Here's how the part is built. I have some questions about the finished solid (model axes, mm). Face numbers are marked on the shaded views. Coordinates: 2 decimals unless noted, no trailing zeros. Write each loop counter-clockwise with the first axis right and the second up, starting at its lowest first coordinate (ties: lowest second). Pieces come first, ordered by that corner, then holes.
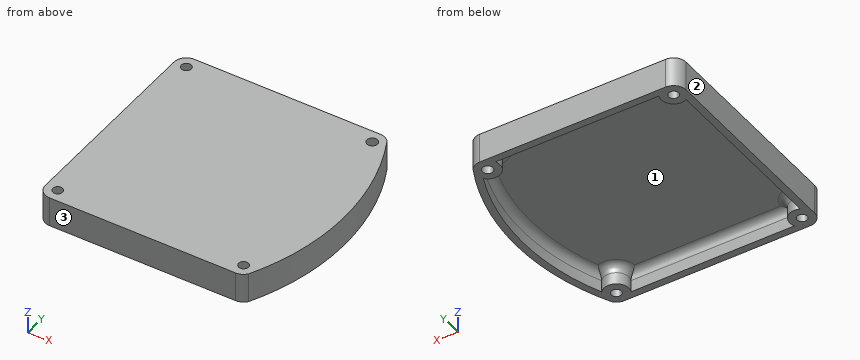
Autodesk Inventor part; units mm, degrees
ref_plane "YZ Plane" through (0, 0, 0) normal (1, 0, 0) x (0, 1, 0)
ref_plane "XZ Plane" through (0, 0, 0) normal (0, 1, 0) x (-1, 0, 0)
ref_plane "XY Plane" through (0, 0, 0) normal (0, 0, 1) x (1, 0, 0)
sketch "Sketch1" plane through (0, 0, 0) normal (0, 0, 1) x (1, 0, 0)
  line L0 (-44.1613, -40) -> (-44.1613, 40)
  arc A0 (-39.1613, 45) -> (-44.1613, 40) centre (-39.1613, 40) ccw
  line L1 (-39.1613, 45) -> (35.8387, 45)
  arc A1 (39.8387, 43) -> (35.8387, 45) centre (35.8387, 40) ccw
  arc A2 (39.8387, -43) -> (39.8387, 43) centre (-44.1612, 0) ccw
  arc A3 (35.8387, -45) -> (39.8387, -43) centre (35.8387, -39.9999) ccw
  line L2 (35.8387, -45) -> (-39.1613, -45)
  arc A4 (-44.1613, -40) -> (-39.1613, -45) centre (-39.1613, -40) ccw
  circle A5 centre (-39.1613, -40) radius 2
  circle A6 centre (-39.1613, 40) radius 2
  circle A7 centre (35.8387, 40) radius 2.15
  circle A8 centre (35.8387, -40) radius 2
  arc A9 (37.5587, 41.29) -> (35.8387, 42.15) centre (35.8387, 40) ccw
  line L3 (35.8387, 42.15) -> (-39.1613, 42.15)
  arc A10 (-39.1613, 42.15) -> (-41.3113, 40) centre (-39.1613, 40) ccw
  line L4 (-41.3113, 40) -> (-41.3113, -40)
  arc A11 (-41.3113, -40) -> (-39.1613, -42.15) centre (-39.1613, -40) ccw
  line L5 (-39.1613, -42.15) -> (35.8387, -42.15)
  arc A12 (35.8387, -42.15) -> (37.5587, -41.29) centre (35.8387, -39.9999) ccw
  arc A13 (37.3698, -41.7362) -> (37.3698, 41.7362) centre (-44.1612, 0) ccw
  circle A14 centre (-39.1613, 40) radius 5
  circle A15 centre (35.8387, 40) radius 5
  circle A16 centre (35.8387, -40) radius 5
  circle A17 centre (-39.1613, -40) radius 5
  point P0 (0, 0)
  point P1 (39.8387, -43)
  point P2 (31.3246, 42.15)
  point P3 (39.7021, 36.826)
  point P4 (39.7021, -36.826)
  point P5 (31.3246, -42.15)
  point P6 (-34.6471, -42.15)
  point P7 (-41.3113, -35.4859)
  point P8 (-41.3113, 35.4859)
  point P9 (-34.6471, 42.15)
extrude "Extrusion1" add sketch "Sketch1" along normal blind 8 contours A17 L4 A11 L5 A4 | L0 A14 L4 A17 | A0 A14 L3 A10 L4 | A17 L5 A16 L2 | A17 L5 A11 L4 | L1 A15 L3 A14 | L4 A10 L3 A14 | A16 A2 A3 | A1 A2 A15 A13 A7 L3 | L3 A7 A13 A15 | A16 A13 A15 A2
sketch "Sketch2" plane through (0, 0, 8) normal (0, 0, 1) x (1, 0, 0)
  arc A0 (-39.1613, 45) -> (-44.1613, 40) centre (-39.1613, 40) ccw
  line L0 (-44.1613, 40) -> (-44.1613, -40)
  arc A1 (-44.1613, -40) -> (-39.1613, -45) centre (-39.1613, -40) ccw
  line L1 (-39.1613, -45) -> (35.8387, -45)
  arc A2 (35.8387, -45) -> (39.8387, -43) centre (35.8387, -39.9999) ccw
  arc A3 (39.8387, -43) -> (39.8387, 43) centre (-44.1612, 0) ccw
  arc A4 (39.8387, 43) -> (35.8387, 45) centre (35.8387, 40) ccw
  line L2 (35.8387, 45) -> (-39.1613, 45)
  circle A5 centre (35.8387, 40) radius 2.15
  circle A6 centre (35.8387, -40) radius 2
  circle A7 centre (-39.1613, -40) radius 2
  circle A8 centre (-39.1613, 40) radius 2
  arc A9 (31.3246, 42.15) -> (39.7021, 36.826) centre (35.8387, 40) ccw
  arc A10 (39.7021, -36.826) -> (39.7021, 36.826) centre (-44.1612, 0) ccw
  arc A11 (39.7021, -36.826) -> (31.3246, -42.15) centre (35.8387, -40) ccw
  line L3 (31.3246, -42.15) -> (-34.6471, -42.15)
  arc A12 (-34.6471, -42.15) -> (-41.3113, -35.4859) centre (-39.1613, -40) ccw
  line L4 (-41.3113, -35.4859) -> (-41.3113, 35.4859)
  arc A13 (-41.3113, 35.4859) -> (-34.6471, 42.15) centre (-39.1613, 40) ccw
  line L5 (-34.6471, 42.15) -> (31.3246, 42.15)
  point P0 (0, 0)
extrude "Extrusion2" add sketch "Sketch2" along normal blind 4 contours L2 A4 A3 A2 L1 A1 L0 A0 | A9 A10 A11 L3 A12 L4 A13 L5
fillet "Fillet1" radius 3.175 8 edges at (-1.6613, 42.15, 8) (-41.3113, 0, 8) (-1.6613, -42.15, 8) (47.4314, 0, 8) (-35.6257, -36.4645, 8) (-35.6257, 36.4645, 8) (33.1569, 35.7801, 8) (33.1569, -35.7801, 8)
properties part number "Bottom Case"
1. Thinking about a two-plate mould opening in X: for the marked faces 1, 2 and 3, which applies, pulls with the +X half, pulls with the -X half, needs draft (parallel to the pull), parting line crosses it, or undercut?
2. For pin 1 Ø5 at (y, z) = (23, 3.5) entering from +X; pin 2 Ø5 at (y, z) = (-27.5, 7) entering from +X; pin 3 Ø1 at (x, y) = (-14.5, -14.5) entering from -Z; pin 4 Ø2.5 at (x, y) = (35.84, -40) entering from -Z, each with a flat end and sliding along its axis, tell me the tip position at first contact or that it passes through.
3. If I drill on line 1 (Y direction, x = -38, z = 7.25); line 2 (Y direction, x = 34, z = 0.5); line 3 (Y direction, x = -5.5, z = 5.75), over which ranges is the centre line in solid material (lowest first)?
4. I want a section at A-A (x = -7). List the corners of the cut face in (y, z) for me (3 decimals), then the cut area to 3 significant figures.
Response values:
1. face 1: undercut
1. face 2: pulls with the -X half
1. face 3: needs draft
2. pin 1: stops at x = 47.95
2. pin 2: stops at x = 46.83
2. pin 3: stops at z = 8
2. pin 4: passes through
3. line 1: y = -45 to -41.63, -38.37 to -33.99, 33.99 to 38.37, 41.63 to 45
3. line 2: y = -45 to -40.79, -39.21 to -35.35, 35.35 to 38.89, 41.11 to 45
3. line 3: y = -45 to -42.01, 42.01 to 45
4. outline: (-45, 0) - (-42.15, 0) - (-42.15, 4.825) arc R3.175 cw to (-38.975, 8) - (38.975, 8) arc R3.175 cw to (42.15, 4.825) - (42.15, 0) - (45, 0) - (45, 12) - (-45, 12) - close
4. area: 410 mm2
